Drawing for the job (mm, zero at the part's lowest x, y, z). A direction names the side the tool comes from. Give positions to 0.01 mm unless a question says otherwise; leave off trailing zeros. Order: outer loops, then holes, each group sorted by start corner. A loop starts at its lowest first (then second) coordinate and runs counter-clockwise, first axis right, second up. Notation, with made-up numbers: (-33.75, 26.5) - (-7.75, 26.5) arc R17 ccw to (-7.75, 44.5) - close; hole circle Ø1 at (2.5, -23). An arc over 180 degrees is marked (long way). Use a Markdown table: item, result. Add a question column.
(1) Which spindle directions (+Z, -Z, +X, -X, +Y, -Y) get a long thin tool onto all of the face, cutting with end or side? Do the marked faces 1 and 2. Say none if no direction does.
(2) Wall check: line 1 (Y direction, x = 15, z = 1.6); line 2 (Y direction, x = 2.4, z = 10); line 3 (X direction, y = 26, z = 18). Give the ranges that are in metal, low to high.
(3) Flat gauge pins, fed straight in: pin 1 (5.5 mm diameter, centred on y = 35, z = 15, fed in from +X); pin 2 (6.5 mm diameter, centred on x = 15, y = 5, fed in from +Z); pin 3 (2.5 mm diameter, centred on x = 15, y = 35, fed in from +Z). Where does each tip first touch, or does it go through?
(4) Slice it at A-A (z = 10). Write the cut outline in (x, y), then the cut area to 3 significant figures.
(5) Slice it at D-D (x = 14.25). Write the cut outline in (y, z).
(6) Slice it at B-B (y = 20). Write the cut outline in (x, z), then the cut area to 3 significant figures.
(7) Slice it at C-C (z = 15). Write the cut outline in (x, y).
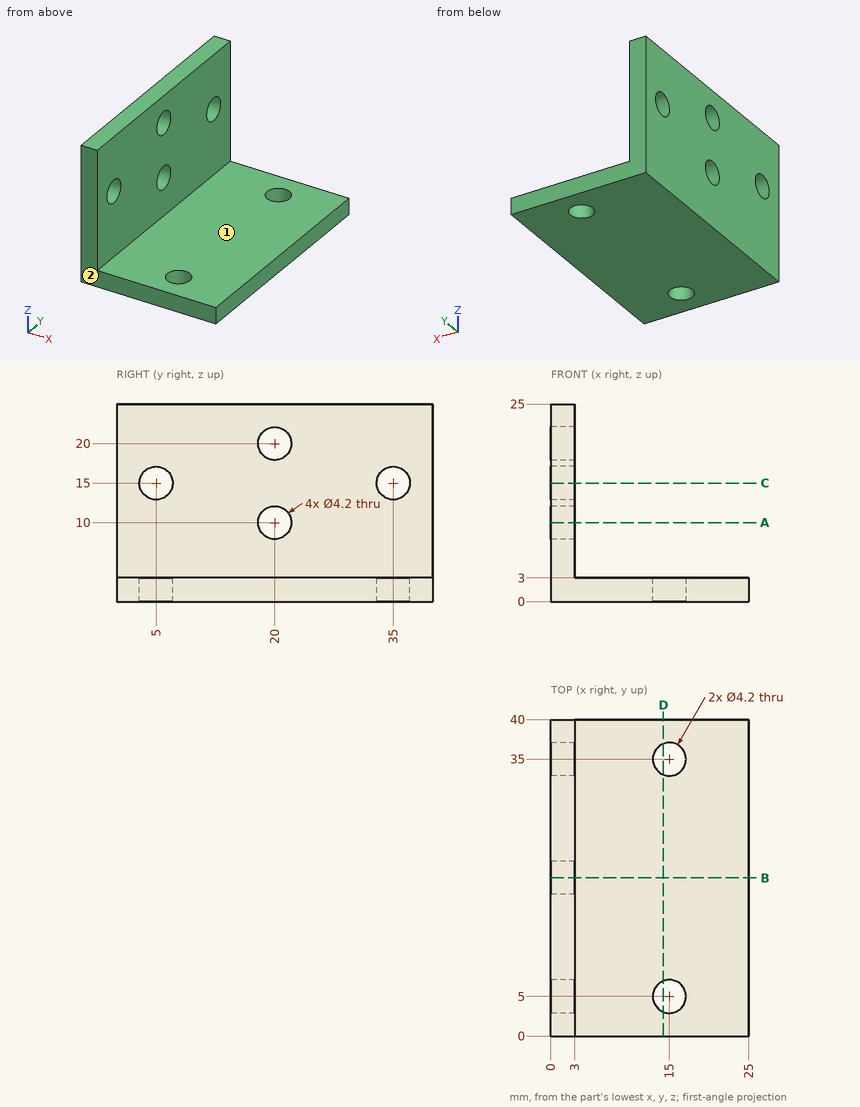
Solution:
| question | item | result |
|---|---|---|
| 1 | face 1 | +Z, +X, +Y, -Y |
| 1 | face 2 | +Z, -Z, +X, -X, -Y |
| 2 | line 1 | 0 to 2.9, 7.1 to 32.9, 37.1 to 40 |
| 2 | line 2 | 0 to 17.9, 22.1 to 40 |
| 2 | line 3 | 0 to 3 |
| 3 | pin 1 | x = 3 |
| 3 | pin 2 | z = 3 |
| 3 | pin 3 | through |
| 4 | outline | (0, 0) - (3, 0) - (3, 17.9) - (0, 17.9) - close; (0, 22.1) - (3, 22.1) - (3, 40) - (0, 40) - close |
| 4 | area | 107 mm2 |
| 5 | outline | (0, 0) - (3.04, 0) - (3.04, 3) - (0, 3) - close; (6.96, 0) - (33.04, 0) - (33.04, 3) - (6.96, 3) - close; (36.96, 0) - (40, 0) - (40, 3) - (36.96, 3) - close |
| 6 | outline | (0, 0) - (25, 0) - (25, 3) - (3, 3) - (3, 7.9) - (0, 7.9) - close; (0, 12.1) - (3, 12.1) - (3, 17.9) - (0, 17.9) - close; (0, 22.1) - (3, 22.1) - (3, 25) - (0, 25) - close |
| 6 | area | 116 mm2 |
| 7 | outline | (0, 0) - (3, 0) - (3, 2.9) - (0, 2.9) - close; (0, 7.1) - (3, 7.1) - (3, 32.9) - (0, 32.9) - close; (0, 37.1) - (3, 37.1) - (3, 40) - (0, 40) - close |
